The figure shows three views and two pictorial views of one solid part (mm, origin at its lowest corner). Answer the questions. Round coordinates to 2 decimals unless told otherwise and drop trailing zeros. Order: outer loops, then holes, each group sorted by start corner. A loop starts at its lowest first (then second) coordinate and runs counter-clockwise, first axis right, second up. Notation, with made-up numbers: (-3, -17) -> (5, -17) arc R14 ccw to (5, 1) -> close; hole circle Ø9 at (-39, -19). An arc over 180 degrees is marked (long way). One line per item, written item: value. Start each with the question number.
1. Section A-A (y = 0.75) is taken. Give the vertices of the cut face in (x, z).
2. Consider line 1 (Y direction, x = 2, z = 0.15) (1 decimal); line 2 (Y direction, x = 1.2, z = 0.1) (1 decimal); line 3 (Y direction, x = 2.2, z = 0.15) (1 decimal). Determine where each line is inside the solid, lowest interval first.
3. Section B-B (z = 0.1) is taken. Give the vertices of the cut face in (x, y).
4. Section D-D (x = 0.7) is taken. Give the vertices of the cut face in (y, z).
5. Section C-C (y = 12) is taken. Give the vertices of the cut face in (x, z).
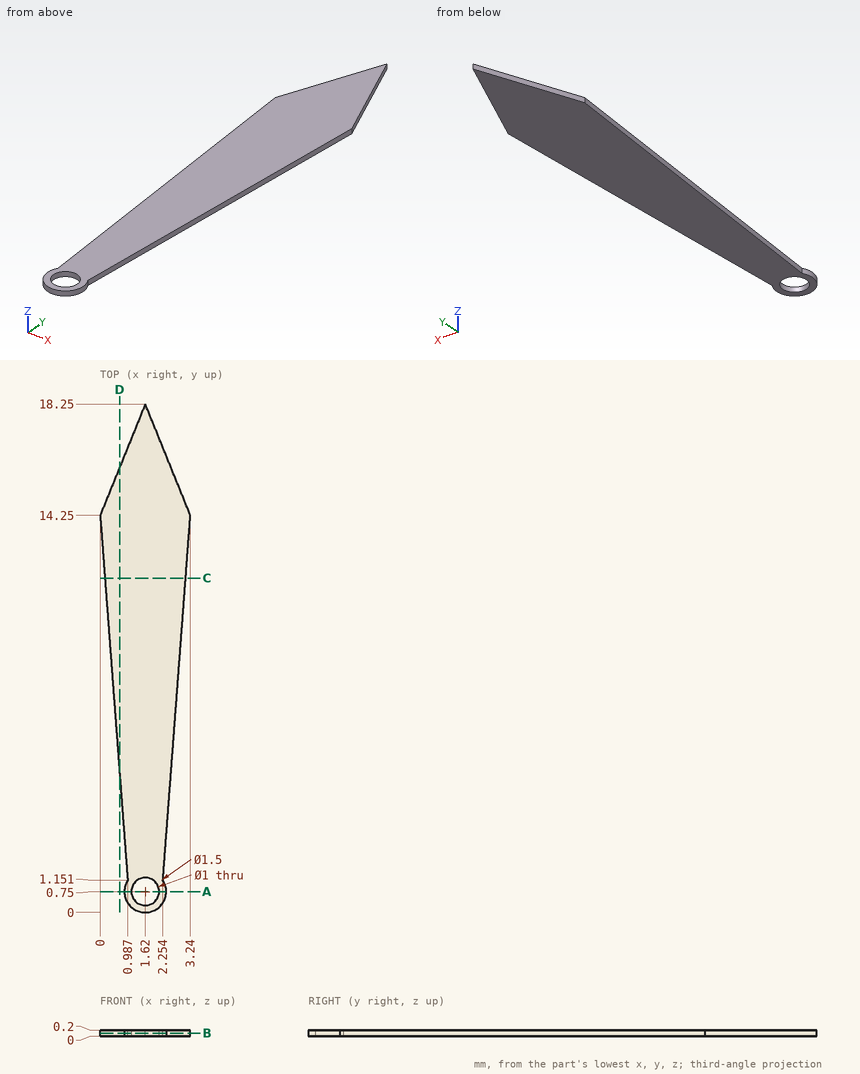
Answer:
1. outline: (0.87, 0) -> (1.12, 0) -> (1.12, 0.2) -> (0.87, 0.2) -> close; (2.12, 0) -> (2.37, 0) -> (2.37, 0.2) -> (2.12, 0.2) -> close
2. line 1: 0.1 to 0.4, 1.1 to 17.3
2. line 2: 0.1 to 0.5, 1 to 17.2
2. line 3: 0.3 to 16.8
3. outline: (0, 14.25) -> (0.99, 1.15) arc R0.75 ccw (long way) to (2.25, 1.15) -> (3.24, 14.25) -> (1.62, 18.25) -> close; hole circle Ø1 at (1.62, 0.75)
4. outline: (4.96, 0) -> (15.98, 0) -> (15.98, 0.2) -> (4.96, 0.2) -> close
5. outline: (0.17, 0) -> (3.07, 0) -> (3.07, 0.2) -> (0.17, 0.2) -> close
